Can you work these out from the model? Positions are in its coordinate system, mm. Give positions to 0.01 mm unless a question says otherwise; leave off trailing zeros. Loops run counter-clockwise (first coordinate to the right, second up) from the corner with the lowest first, then second, coordinate; pieces in that order, holes last. Notation, with made-up numbers: (37, 9) - (91, 9) arc R25 ccw to (91, 36) - close; hole circle Ø2 at (9.25, 72). An arc over 180 degrees is marked (long way). Write item = value, one per line.
Autodesk Inventor part; units mm, degrees
ref_plane "YZ Plane" through (0, 0, 0) normal (1, 0, 0) x (0, 1, 0)
ref_plane "XZ Plane" through (0, 0, 0) normal (0, 1, 0) x (-1, 0, 0)
ref_plane "XY Plane" through (0, 0, 0) normal (0, 0, 1) x (1, 0, 0)
sketch "Sketch1" plane through (0, 0, 0) normal (0, 0, 1) x (1, 0, 0)
  line L0 (-250, 0) -> (0, 0) construction
  line L1 (-250, -50) -> (0, -50)
  line L2 (0, 50) -> (-250, 50)
  arc A0 (-250, 50) -> (-250, -50) centre (-250, 0) ccw
  line L3 (0, 50) -> (0, -50)
  circle A1 centre (-250, 0) radius 25
  circle A2 centre (-125, 0) radius 25
  circle A3 centre (0, 0) radius 25
  point P0 (-125, 0)
  point P1 (0, -25)
  point P2 (0, 25)
  dimension "d2" = 250
  dimension "d3" = 50
  dimension "d4" = 50
  dimension "d6" = 125
  dimension "d7" = 125
extrude "Extrusion1" add sketch "Sketch1" along normal mid plane 20 contours A0 L2 L3 A3 L1
properties part number "CE-10.2.1.2" material "Aluminum 6061"
Q1. Imagine slicing it at C-C, the plane z = 6.25. Write out the boundary of the cut face in (x, y), then the cut area to 3 significant figures.
Output:
outline = (-250, -50) - (0, -50) - (0, -25) arc R25 cw to (0, 25) - (0, 50) - (-250, 50) arc R50 ccw to start; hole circle Ø50 at (-250, 0); hole circle Ø50 at (-125, 0)
area = 24,000 mm2
Q2. Imagine slicing it at D-D, the plane y = -22. Write out the boundary of the cut face in (x, z).
Output:
outline = (-294.9, -10) - (-261.87, -10) - (-261.87, 10) - (-294.9, 10) - close; (-238.13, -10) - (-136.87, -10) - (-136.87, 10) - (-238.13, 10) - close; (-113.13, -10) - (-11.87, -10) - (-11.87, 10) - (-113.13, 10) - close
Q3. For pin 1 (6 mm diameter, centred on y = -28, z = -6, fed in from -X); pin 2 (12 mm diameter, centred on y = 8.5, z = 2, fed in from -X); pin 3 (2 mm diameter, centred on y = 40, z = 7, fed in from -X), each with a flat end and sliding along its axis, tell me the tip position at first contact or that it passes through.
Output:
pin_1 = -293.3
pin_2 = -299.94
pin_3 = -281.29
Q4. Imagine slicing it at A-A, the plane y = 0. Write out the boundary of the cut face in (x, z).
Output:
outline = (-300, -10) - (-275, -10) - (-275, 10) - (-300, 10) - close; (-225, -10) - (-150, -10) - (-150, 10) - (-225, 10) - close; (-100, -10) - (-25, -10) - (-25, 10) - (-100, 10) - close
Q5. I need wall thicknesses on L1, parallel to Y at x = -250, z = -2.25; L2, parallel to X at y = -20, z = -9; L3, parallel to X at y = -4.5, z = 5. Which ranges of each line are inside material? Lowest first, please.
Output:
L1 = -50 to -25, 25 to 50
L2 = -295.83 to -265, -235 to -140, -110 to -15
L3 = -299.8 to -274.59, -225.41 to -149.59, -100.41 to -24.59
Q6. Imagine slicing it at B-B, the plane x = -267. Write out the boundary of the cut face in (y, z), then the cut area to 3 significant figures.
Output:
outline = (-47.02, -10) - (-18.33, -10) - (-18.33, 10) - (-47.02, 10) - close; (18.33, -10) - (47.02, -10) - (47.02, 10) - (18.33, 10) - close
area = 1,150 mm2
Q7. We'd pull the mould along Y, two halves only. Please class faces 1 (the flat face through (0, -37, 0)), 2 (the cylindrical face through (-226.154, -7.509, -0.14)), 3 (the flat face through (-127, -50, 0)), 4 (the cylindrical face through (-299.988, -1.099, -0.14)): released by +Y, released by -Y, zero draft, split by the parting line, or undercut.
Output:
face_1 = zero draft
face_2 = undercut
face_3 = released by -Y
face_4 = split by the parting line
